from build123d import *

# Parameters (mm, degrees)
MODEL_R             = 5.5
MODEL_R_2           = 2.75
BOSS_EXTRUDE1_DEPTH = 6.6


with BuildPart() as part:
    # Model → Boss-Extrude1 (new body)
    with BuildSketch(Plane.XY):
        with BuildLine():
            Line((146.910001664, 29.054806781), (156.910001664, 19.054806781))
            Line((156.910001664, 19.054806781), (156.910001664, 15))
            Line((156.910001664, 15), (171.910001664, 0))
            Line((171.910001664, 0), (187.8, 0))
            Line((187.8, 0), (187.8, 14.95))
            Line((187.8, 14.95), (176.8, 14.95))
            Line((176.8, 14.95), (176.8, 13.365))
            ThreePointArc((176.8, 13.365), (176.653553391, 13.011446609), (176.3, 12.865))
            Line((176.3, 12.865), (172.3, 12.865))
            ThreePointArc((172.3, 12.865), (171.946446609, 13.011446609), (171.8, 13.365))
            Line((171.8, 13.365), (171.8, 14.95))
            Line((171.8, 14.95), (167.3, 14.95))
            ThreePointArc((167.3, 14.95), (166.946446609, 15.096446609), (166.8, 15.45))
            Line((166.8, 15.45), (166.8, 18))
            ThreePointArc((166.8, 18), (166.946446609, 18.353553391), (167.3, 18.5))
            Line((167.3, 18.5), (171.8, 18.5))
            Line((171.8, 18.5), (171.8, 20.085))
            ThreePointArc((171.8, 20.085), (171.946446609, 20.438553391), (172.3, 20.585))
            Line((172.3, 20.585), (176.3, 20.585))
            ThreePointArc((176.3, 20.585), (176.653553391, 20.438553391), (176.8, 20.085))
            Line((176.8, 20.085), (176.8, 18.5))
            Line((176.8, 18.5), (187.8, 18.5))
            Line((187.8, 18.5), (187.8, 37.5))
            Line((187.8, 37.5), (191.8, 37.5))
            ThreePointArc((191.8, 37.5), (193.567766953, 38.232233047), (194.3, 40))
            Line((194.3, 40), (194.3, 50))
            ThreePointArc((194.3, 50), (193.567766953, 51.767766953), (191.8, 52.5))
            Line((191.8, 52.5), (187.8, 52.5))
            Line((187.8, 52.5), (187.8, 71.5))
            Line((187.8, 71.5), (176.8, 71.5))
            Line((176.8, 71.5), (176.8, 69.915))
            ThreePointArc((176.8, 69.915), (176.653553391, 69.561446609), (176.3, 69.415))
            Line((176.3, 69.415), (172.3, 69.415))
            ThreePointArc((172.3, 69.415), (171.946446609, 69.561446609), (171.8, 69.915))
            Line((171.8, 69.915), (171.8, 71.5))
            Line((171.8, 71.5), (167.3, 71.5))
            ThreePointArc((167.3, 71.5), (166.946446609, 71.646446609), (166.8, 72))
            Line((166.8, 72), (166.8, 74.55))
            ThreePointArc((166.8, 74.55), (166.946446609, 74.903553391), (167.3, 75.05))
            Line((167.3, 75.05), (171.8, 75.05))
            Line((171.8, 75.05), (171.8, 76.635))
            ThreePointArc((171.8, 76.635), (171.946446609, 76.988553391), (172.3, 77.135))
            Line((172.3, 77.135), (176.3, 77.135))
            ThreePointArc((176.3, 77.135), (176.653553391, 76.988553391), (176.8, 76.635))
            Line((176.8, 76.635), (176.8, 75.05))
            Line((176.8, 75.05), (187.8, 75.05))
            Line((187.8, 75.05), (187.8, 88))
            Line((187.8, 88), (185.8, 90))
            Line((185.8, 90), (113.770001664, 90))
            Line((113.770001664, 90), (113.770001664, 77.3))
            Line((113.770001664, 77.3), (106.910001664, 77.3))
            Line((106.910001664, 77.3), (106.910001664, 90))
            Line((106.910001664, 90), (81.510001665, 90))
            Line((81.510001665, 90), (81.510001665, 77.3))
            Line((81.510001665, 77.3), (74.650001665, 77.3))
            Line((74.650001665, 77.3), (74.650001665, 90))
            Line((74.650001665, 90), (2, 90))
            Line((2, 90), (0, 88))
            Line((0, 88), (0, 75.05))
            Line((0, 75.05), (11, 75.05))
            Line((11, 75.05), (11, 76.635))
            ThreePointArc((11, 76.635), (11.146446609, 76.988553391), (11.5, 77.135))
            Line((11.5, 77.135), (15.5, 77.135))
            ThreePointArc((15.5, 77.135), (15.853553391, 76.988553391), (16, 76.635))
            Line((16, 76.635), (16, 75.05))
            Line((16, 75.05), (20.5, 75.05))
            ThreePointArc((20.5, 75.05), (20.853553391, 74.903553391), (21, 74.55))
            Line((21, 74.55), (21, 72))
            ThreePointArc((21, 72), (20.853553391, 71.646446609), (20.5, 71.5))
            Line((20.5, 71.5), (16, 71.5))
            Line((16, 71.5), (16, 69.915))
            ThreePointArc((16, 69.915), (15.853553391, 69.561446609), (15.5, 69.415))
            Line((15.5, 69.415), (11.5, 69.415))
            ThreePointArc((11.5, 69.415), (11.146446609, 69.561446609), (11, 69.915))
            Line((11, 69.915), (11, 71.5))
            Line((11, 71.5), (0, 71.5))
            Line((0, 71.5), (0, 52.5))
            Line((0, 52.5), (-4, 52.5))
            ThreePointArc((-4, 52.5), (-5.767766953, 51.767766953), (-6.5, 50))
            Line((-6.5, 50), (-6.5, 40))
            ThreePointArc((-6.5, 40), (-5.767766953, 38.232233047), (-4, 37.5))
            Line((-4, 37.5), (0, 37.5))
            Line((0, 37.5), (0, 18.5))
            Line((0, 18.5), (11, 18.5))
            Line((11, 18.5), (11, 20.085))
            ThreePointArc((11, 20.085), (11.146446609, 20.438553391), (11.5, 20.585))
            Line((11.5, 20.585), (15.5, 20.585))
            ThreePointArc((15.5, 20.585), (15.853553391, 20.438553391), (16, 20.085))
            Line((16, 20.085), (16, 18.5))
            Line((16, 18.5), (20.5, 18.5))
            ThreePointArc((20.5, 18.5), (20.853553391, 18.353553391), (21, 18))
            Line((21, 18), (21, 15.45))
            ThreePointArc((21, 15.45), (20.853553391, 15.096446609), (20.5, 14.95))
            Line((20.5, 14.95), (16, 14.95))
            Line((16, 14.95), (16, 13.365))
            ThreePointArc((16, 13.365), (15.853553391, 13.011446609), (15.5, 12.865))
            Line((15.5, 12.865), (11.5, 12.865))
            ThreePointArc((11.5, 12.865), (11.146446609, 13.011446609), (11, 13.365))
            Line((11, 13.365), (11, 14.95))
            Line((11, 14.95), (0, 14.95))
            Line((0, 14.95), (0, 0))
            Line((0, 0), (16.510001665, 0))
            Line((16.510001665, 0), (31.510001665, 15))
            Line((31.510001665, 15), (31.510001665, 19.054806781))
            Line((31.510001665, 19.054806781), (41.510001665, 29.054806781))
            Line((41.510001665, 29.054806781), (79.010001665, 29.054806781))
            ThreePointArc((79.010001665, 29.054806781), (80.777768618, 29.787039828), (81.510001665, 31.554806781))
            Line((81.510001665, 31.554806781), (81.510001665, 54.45480678))
            Line((81.510001665, 54.45480678), (106.910001664, 54.45480678))
            Line((106.910001664, 54.45480678), (106.910001664, 31.554806781))
            ThreePointArc((106.910001664, 31.554806781), (107.642234711, 29.787039828), (109.410001664, 29.054806781))
            Line((109.410001664, 29.054806781), (146.910001664, 29.054806781))
        make_face()
        with Locations((139.852001664, 41.754806781)):
            Circle(MODEL_R, mode=Mode.SUBTRACT)
        with Locations((48.568001665, 41.754806781)):
            Circle(MODEL_R, mode=Mode.SUBTRACT)
        with Locations((182.8, 42.08)):
            Circle(MODEL_R_2, mode=Mode.SUBTRACT)
        with Locations((5.62000333, 42.08)):
            Circle(MODEL_R_2, mode=Mode.SUBTRACT)
    extrude(amount=BOSS_EXTRUDE1_DEPTH)


solid = part.part
Design review of the part built by this model. Coordinates are the model's own, in mm. A direction names the side the tool comes from. Give positions to 0.01 mm unless a question says otherwise; leave off trailing zeros. Order: outer loops, then holes, each group sorted by start corner. A loop starts at its lowest first (then second) coordinate and runs counter-clockwise, first axis right, second up. Notation, with made-up numbers: (17, 72.25) - (28, 72.25) arc R27 ccw to (28, 92.25) - close; hole circle Ø2 at (54, -20.75). An arc over 180 degrees is marked (long way). Write item = value, one per line. Start each with the question number.
Q1. We need section C-C on z = 5. State how many separate pieces and enclosed holes the cut face has, plus the area to 3 significant figures.
Q2. We need section D-D on x = 23.5. State the section outline as (y, z) points, plus the area to 3 significant figures.
Q3. We need section B-B on x = 138.5. State the section outline as (y, z) points, plus the area to 3 significant figures.
Q4. We need section A-A on x = 182.8. State the section outline as (y, z) points.
Q5. To check wall thickness, follow L1, parallel to X at y = 83.5, z = 2.75; L2, parallel to Y at x = 182.8, z = 2.75; L3, parallel to X at y = 42.5, z = 4.75. State the ranges of each line that lie inside material, in increasing order. Write a range as from..to.
Q6. Mouldability with a two-part tool opening along X and no side actions: class faces 1 (the face through (81.51, 43, 3)), 2 (the face through (0, 8, 3)), 3 (the face through (6, 14.95, 3)) as released by +X, released by -X, zero draft, split by the parting line, or undercut.
Q7. Tool access review of faces 4 (the face through (170, 71.5, 3)), 5 (the face through (174, 12.865, 3)), 6 (the face through (5, 18.5, 3)), 7 (the face through (190, 52.5, 3)), 8 (the face through (151.84, 24.125, 3.254)): name each direction out of +Z, -Z, +X, -X, +Y, -Y from which nothing blocks a thin tool from reaching the whole face with its end or side.
Q8. Clearance check with flat-ended pins moving along their axes: pin 1 Ø2 at (x, z) = (183, 3.5) entering from -Y; pin 2 Ø2 at (x, z) = (-1.5, 4) entering from -Y; pin 3 Ø2 at (y, z) = (84, 4.5) entering from +X; pin 4 Ø3.5 at (x, z) = (77.5, 2.5) entering from +Y. State where each tip first meets the part, or that it passes through.
Working result:
q1.separate_pieces = 1
q1.enclosed_holes = 4
q1.area = 11,900 mm²
q2.outline = (6.99, 0) - (90, 0) - (90, 6.6) - (6.99, 6.6) - close
q2.area = 548 mm²
q3.outline = (29.05, 0) - (36.42, 0) - (36.42, 6.6) - (29.05, 6.6) - close; (47.09, 0) - (90, 0) - (90, 6.6) - (47.09, 6.6) - close
q3.area = 332 mm²
q4.outline = (0, 0) - (14.95, 0) - (14.95, 6.6) - (0, 6.6) - close; (18.5, 0) - (39.33, 0) - (39.33, 6.6) - (18.5, 6.6) - close; (44.83, 0) - (71.5, 0) - (71.5, 6.6) - (44.83, 6.6) - close; (75.05, 0) - (90, 0) - (90, 6.6) - (75.05, 6.6) - close
q5.L1 = 0..74.65, 81.51..106.91, 113.77..187.8
q5.L2 = 0..14.95, 18.5..39.33, 44.83..71.5, 75.05..90
q5.L3 = -6.5..2.9, 8.34..43.12, 54.02..81.51, 106.91..134.4, 145.3..180.08, 185.52..194.3
q6.face_1 = undercut
q6.face_2 = released by -X
q6.face_3 = zero draft
q7.face_4 = +Z, -Z, +X
q7.face_5 = +Z, -Z
q7.face_6 = +Z, -Z, -X
q7.face_7 = +Z, -Z, +X, +Y
q7.face_8 = +Z, -Z, -Y
q8.pin_1 = 0
q8.pin_2 = 37.5
q8.pin_3 = 187.8
q8.pin_4 = 77.3
